```python
from build123d import *

# Parameters (mm, degrees)
SKETCH1_R           = 5.715
BOSS_EXTRUDE1_DEPTH = 25.4
SKETCH2_R           = 1.5875
BOSS_EXTRUDE2_DEPTH = 5.08
SKETCH4_R           = 1.5875
CUT_EXTRUDE2_DEPTH  = 6.35
SKETCH3_R           = 1.5875
CUT_EXTRUDE3_DEPTH  = 12.43


with BuildPart() as part:
    # Sketch1 → Boss-Extrude1 (new body)
    with BuildSketch(Plane(origin=(0, 0, 0), x_dir=(1, 0, 0), z_dir=(0, 1, 0))):
        Circle(SKETCH1_R)
    extrude(amount=BOSS_EXTRUDE1_DEPTH)

    # Sketch2 → Boss-Extrude2 (add)
    with BuildSketch(Plane(origin=(0, 25.4, 0), x_dir=(1, 0, 0), z_dir=(0, 1, 0))):
        Circle(SKETCH2_R)
    extrude(amount=BOSS_EXTRUDE2_DEPTH)

    # Sketch4 → Cut-Extrude2 (cut)
    with BuildSketch(Plane.XZ):
        Circle(SKETCH4_R)
    extrude(amount=-CUT_EXTRUDE2_DEPTH, mode=Mode.SUBTRACT)

    # Sketch3 → Cut-Extrude3 (cut, through all)
    with BuildSketch(Plane.XY.offset(5.715)):
        with Locations((0, 6.35)):
            Circle(SKETCH3_R)
    extrude(amount=-CUT_EXTRUDE3_DEPTH, mode=Mode.SUBTRACT)


solid = part.part
```
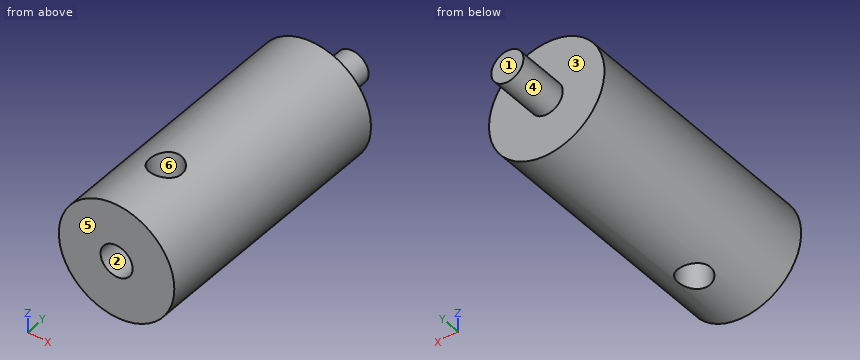
Input: part model. Units: mm. Frame: model coordinates. Face numbers are marked on the shaded views. A direction names the side the tool comes from. Coordinates: 2 decimals unless noted, no trailing zeros. Write each loop counter-clockwise with the first axis right and the second up, starting at its lowest first coordinate (ties: lowest second). Pieces come first, ordered by that corner, then holes. Notation, with made-up numbers: M 82,-5 L 117,-5 A19 cw 117,24 Z; hole C -14,3.5 d9. An arc over 180 degrees is marked long. Use one line per item in the form item = value.
Q1. Draft query along X for the marked faces 4, 5 and 6. Return one class per face: released by +X, released by -X, zero draft, split by the parting line, or undercut.
Answer below:
face_4 = split by the parting line
face_5 = zero draft
face_6 = undercut
Q2. First-contact query: pin 1 (2 mm diameter, centred on x = -1, z = 3, fed in from +Y); pin 2 (4 mm diameter, centred on y = 3.5, z = -3, fed in from +X). Flat tips, straight axial feed; report the tip coordinate or a pass-through.
Answer below:
pin_1 = 25.4
pin_2 = 5.63
Q3. Section A-A (x = 0). Return loops of the section in (y, z) (1 decimal), plus the area to 3 significant figures.
Answer below:
outline = M 0,-5.7 L 4.8,-5.7 L 4.8,-1.6 L 0,-1.6 Z; M 0,1.6 L 4.8,1.6 L 4.8,5.7 L 0,5.7 Z; M 7.9,-5.7 L 25.4,-5.7 L 25.4,-1.6 L 30.5,-1.6 L 30.5,1.6 L 25.4,1.6 L 25.4,5.7 L 7.9,5.7 Z
area = 255 mm²
Q4. Material intervals for probe 1 along Y at (x, z) = (0, 2.75); probe 2 along Z at (x, y) = (0, 4) (1 decimal); probe 3 along Y at (x, z) = (3.5, -1), sorted ascending. Write a range as from..to.
Answer below:
probe_1 = 0..4.76, 7.94..25.4
probe_2 = -5.7..-1.6, 1.6..5.7
probe_3 = 0..25.4
Q5. Section C-C (y = 2). Return loops of the section in (x, z) (1 decimal), plus the area to 3 significant figures.
Answer below:
outline = C 0,0 d11.4; hole C 0,0 d3.2
area = 94.7 mm²
Q6. Set-up query: the marked faces 1, 2 and 3. Return all of +Z, -Z, +X, -X, +Y, -Y with unobstructed straight access to the full face (end or side cutting, diameter ignored); none if empty.
Answer below:
face_1 = +Z, -Z, +X, -X, +Y
face_2 = -Y
face_3 = +Y
